from build123d import *

# Parameters (mm, degrees)
SKETCH1_W           = 200
SKETCH1_H           = 6
SKETCH2_R           = 7
BOSS_EXTRUDE1_DEPTH = 5


with BuildPart() as part:
    # Sketch1 → Revolve1 (revolve)
    with BuildSketch(Plane(origin=(0, 0, 0), x_dir=(1, 0, 0), z_dir=(0, 1, 0)), mode=Mode.PRIVATE) as revolve1_sk:
        with Locations((65.279538905, 9)):
            Rectangle(SKETCH1_W, SKETCH1_H)
    revolve(revolve1_sk.sketch.rotate(Axis((-34.720461095, 0, -6), (1, 0, 0)), 180), axis=Axis((-34.720461095, 0, -6), (1, 0, 0)))

    # Sketch2 → Boss-Extrude1 (add)
    with BuildSketch(Plane.ZY.offset(34.720461095)):
        with Locations((-6, 0)):
            Circle(SKETCH2_R)
    boss_extrude1 = extrude(amount=BOSS_EXTRUDE1_DEPTH)

    # Mirror1: Boss-Extrude1 across plane
    add(boss_extrude1.mirror(Plane(origin=(65.279538905, 0, 0), x_dir=(0, 0, 1), z_dir=(1, 0, 0))))


solid = part.part
Verification items for the finished model (mm, model axes). A direction names the side the tool comes from. Coordinates: 2 decimals unless noted, no trailing zeros. Write each loop counter-clockwise with the first axis right and the second up, starting at its lowest first coordinate (ties: lowest second). Pieces come first, ordered by that corner, then holes. Notation, with made-up numbers: (31.25, 74.25) -> (86.25, 74.25) arc R27 cw to (86.25, 111.25) -> close; hole circle Ø9 at (56, 68). An arc over 180 degrees is marked (long way). One line per item, written item: value. Start each with the question number.
Q1. Mould release check, pull along X, two halves, no side actions. Record for faces 3 (the cylindrical face through (-37.185, 2.103, 0.677)), 4 (the flat face through (170.28, 0, -6)), 5 (the flat face through (165.28, 2, 0)): pulls with the +X half, pulls with the -X half, needs draft (parallel to the pull), parting line crosses it, or undercut.
Q2. Cross-section at A-A on y = 0. Enter the section's corners in (x, z), and give its area (3 significant figures).
Q3. Thickness scan on L1, parallel to X at y = -4.25, z = -10.5; L2, parallel to Y at x = 60, z = -6; L3, parallel to Z at x = 145, y = 2.75. Record the ranges inside material, lowest first. Write a range as from..to.
Q4. Cross-section at B-B on z = -6. Enter the section's corners in (x, y), and give its area (3 significant figures).
Q5. Cross-section at C-C on x = -14.5. Enter the section's corners in (y, z), and give its area (3 significant figures).
Q6. Go/stop test with flat-tipped pins: P1, Ø1.5, axis at x = 2.5, z = -10.5, coming from the -Y side; P2, Ø1.5, axis at x = -3.5, z = -4.5, coming from the -Y side; P3, Ø1.5, axis at x = 112, z = -7, coming from the +Y side. Record where each tip stops, or that it passes through.
Q7. Access from +Z, -Z, +X, -X, +Y, -Y to the whole of each face (thin tool, end or side, straight path). Record for faces 1 (the flat face through (-39.72, 0, -6)), 2 (the cylindrical face through (66.68, -4.06, -10.42)).
Checked values:
1. face 3: needs draft
1. face 4: pulls with the +X half
1. face 5: undercut
2. outline: (-39.72, -13) -> (-34.72, -13) -> (-34.72, -12) -> (165.28, -12) -> (165.28, -13) -> (170.28, -13) -> (170.28, 1) -> (165.28, 1) -> (165.28, 0) -> (-34.72, 0) -> (-34.72, 1) -> (-39.72, 1) -> close
2. area: 2,540 mm²
3. L1: x = -39.72..-34.72, 165.28..170.28
3. L2: y = -6..6
3. L3: z = -11.33..-0.67
4. outline: (-39.72, -7) -> (-34.72, -7) -> (-34.72, -6) -> (165.28, -6) -> (165.28, -7) -> (170.28, -7) -> (170.28, 7) -> (165.28, 7) -> (165.28, 6) -> (-34.72, 6) -> (-34.72, 7) -> (-39.72, 7) -> close
4. area: 2,540 mm²
5. outline: circle Ø12 at (0, -6)
5. area: 113 mm²
6. P1: stops at y = -4.68
6. P2: stops at y = -5.95
6. P3: stops at y = 5.99
7. face 1: +Z, -Z, -X, +Y, -Y
7. face 2: none
